Source: CAD feature listing. Evaluate the final solid. Frame: model axes, mm. Coordinates: 2 decimals unless noted, no trailing zeros. Loops run counter-clockwise (first coordinate to the right, second up) from the corner with the lowest first, then second, coordinate; pieces in that order, holes last. Notation, with made-up numbers: (40, -30) -> (81, -30) arc R28 cw to (81, -9) -> close; hole circle Ø11 at (10.5, 86). An arc over 180 degrees is marked (long way). Answer as CSV lines item,"result".
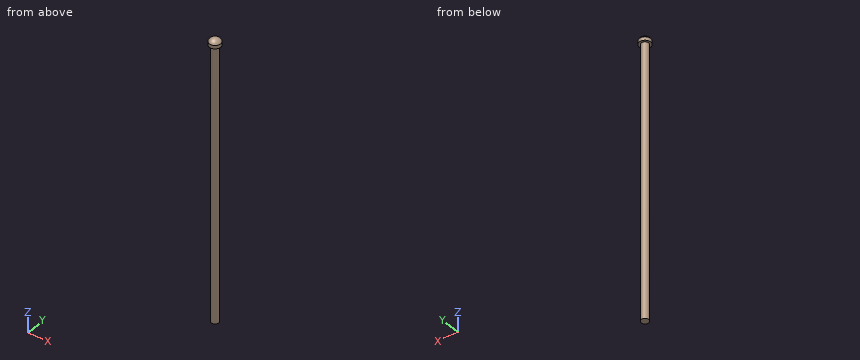
from build123d import *

# Parameters (mm, degrees)
SKETCH_1_R         = 3.25
SKETCH_3_R         = 5
EXTRUDE_1_DEPTH    = 3
DOME_1_FACE_RADIUS = 5
DOME_1_HEIGHT      = 3


with BuildPart() as part:
    # По траектории1: sweep along a path in Эскиз2
    with BuildLine(Plane(origin=(0, 0, -120), x_dir=(0, 0, -1), z_dir=(1, 0, 0))) as sweep_1_path:
        Line((-120, 0), (120, 0))
    # Эскиз1 → По траектории1 (sweep)
    with BuildSketch(Plane.XY):
        with Locations((5, 60)):
            Circle(SKETCH_1_R)
    sweep(path=sweep_1_path.line)

    # Эскиз3 → Бобышка-Вытянуть1 (add)
    with BuildSketch(Plane.XY):
        with Locations((5, 60)):
            Circle(SKETCH_3_R)
    extrude(amount=EXTRUDE_1_DEPTH)

    # Купол1: a dome of height H over a round flat face of radius A is a cap of a sphere of radius (A * A + H * H) / (2 * H)
    dome_1_r = (DOME_1_FACE_RADIUS * DOME_1_FACE_RADIUS + DOME_1_HEIGHT * DOME_1_HEIGHT) / (2 * DOME_1_HEIGHT)
    dome_1_base = Plane((5, 60, 3), z_dir=(0, 0, 1))
    with Locations(dome_1_base.offset(DOME_1_HEIGHT - dome_1_r)):
        dome_1_ball = Sphere(dome_1_r, mode=Mode.PRIVATE)
    add(split(dome_1_ball, bisect_by=dome_1_base, keep=Keep.TOP, mode=Mode.PRIVATE))


solid = part.part
(1) Cut plane B-B (x = 5). Return the cut outline in (y, z).
Computed values:
outline,"(55, 0) -> (56.75, 0) -> (56.75, -240) -> (63.25, -240) -> (63.25, 0) -> (65, 0) -> (65, 3) arc R5.67 ccw to (55, 3) -> close"
(2) Cut plane C-C (z = -38). Return the cut outline in (x, y).
Computed values:
outline,"circle Ø6.5 at (5, 60)"
(3) Material intervals for L1, parallel to Z at x = 5.5, y = 59.75; L2, parallel to Y at x = 5, z = -209; L3, parallel to Z at x = 6, y = 63.5, sorted ascending. Write a range as [from, to].
Computed values:
L1,"[-240, 5.97]"
L2,"[56.75, 63.25]"
L3,"[0, 4.68]"
(4) Pin query (flat end, axial travel): pin 1 Ø1.5 at (x, z) = (2.5, -154.5) entering from +Y; pin 2 Ø1 at (y, z) = (58.5, -195) entering from +X; pin 3 Ø4 at (x, z) = (4.5, -214) entering from +Y. Return the tip coordinate at first contact, or that it passes through.
Computed values:
pin 1,"y = 62.74"
pin 2,"x = 8.09"
pin 3,"y = 63.25"
(5) Cut plane A-A (y = 60). Return the cut outline in (x, z), then the cut area to 3 significant figures.
Computed values:
outline,"(0, 0) -> (1.75, 0) -> (1.75, -240) -> (8.25, -240) -> (8.25, 0) -> (10, 0) -> (10, 3) arc R5.67 ccw to (0, 3) -> close"
area,"1,610 mm^2"
